For this review, take the finished solid that the model builds, in its own axes (mm). Face numbers are marked on the shaded views. A direction names the side the tool comes from. Round coordinates to 2 decimals unless told otherwise and drop trailing zeros. Order: outer loops, then holes, each group sorted by start corner. A loop starts at its lowest first (then second) coordinate and runs counter-clockwise, first axis right, second up.
```python
from build123d import *

# Parameters (mm, degrees)
SKETCH1_W               = 69.85
SKETCH1_H               = 29.464
BOSS_EXTRUDE1_DEPTH     = 16.764
SKETCH2_W               = 25.4
SKETCH2_H               = 6.35
CUT_EXTRUDE1_DEPTH      = 69.85
SKETCH3_W               = 25.4
SKETCH3_H               = 6.35
CUT_EXTRUDE2_DEPTH      = 50.8
SKETCH5_W               = 61.722
SKETCH5_H               = 17.1196
CUT_EXTRUDE3_DEPTH      = 1.016
SKETCH5_3_R             = 0.81915
CUT_EXTRUDE4_DEPTH      = 42.446581825
SKETCH7_W               = 69.85
SKETCH7_H               = 7.62
BOSS_EXTRUDE2_DEPTH     = 25.4
CUT_EXTRUDE9_DEPTH      = 74.328616651
CUT_EXTRUDE9_DEPTH_BACK = 74.328616651
SKETCH13_R              = 2.7051
CUT_EXTRUDE12_DEPTH     = 4.064
SKETCH17_W              = 1.905
SKETCH17_H              = 6.477
CUT_EXTRUDE13_DEPTH     = 25.4
FILLET1_R               = 7.62


with BuildPart() as part:
    # Sketch1 → Boss-Extrude1 (new body)
    with BuildSketch(Plane(origin=(0, 0, 0), x_dir=(1, 0, 0), z_dir=(0, 1, 0))):
        Rectangle(SKETCH1_W, SKETCH1_H)
    extrude(amount=BOSS_EXTRUDE1_DEPTH)

    # Sketch2 → Cut-Extrude1 (cut)
    with BuildSketch(Plane.ZY.offset(34.925)):
        with Locations((-2.032, 7.239)):
            Rectangle(SKETCH2_W, SKETCH2_H)
    extrude(amount=-CUT_EXTRUDE1_DEPTH, mode=Mode.SUBTRACT)

    # Sketch3 → Cut-Extrude2 (cut)
    with BuildSketch(Plane.ZY.offset(34.925)):
        with Locations((-2.032, 13.589)):
            Rectangle(SKETCH3_W, SKETCH3_H)
    cut_extrude2 = extrude(amount=-CUT_EXTRUDE2_DEPTH, mode=Mode.SUBTRACT)

    # Mirror1: Cut-Extrude2 across plane
    add(cut_extrude2.mirror(Plane(origin=(0, 0, 0), x_dir=(0, 0, 1), z_dir=(1, 0, 0))), mode=Mode.SUBTRACT)

    # Sketch5 → Cut-Extrude3 (cut)
    with BuildSketch(Plane.XZ):
        with Locations((0, 6.1722)):
            Rectangle(SKETCH5_W, SKETCH5_H)
    extrude(amount=-CUT_EXTRUDE3_DEPTH, mode=Mode.SUBTRACT)

    # Sketch5<3> → Cut-Extrude4 (cut, through all)
    with BuildSketch(Plane.XZ):
        with Locations(Location((-27.9908, 0.1524, 0), (0, 0, 270))):
            Circle(SKETCH5_3_R)
        with Locations(Location((27.9908, 0.1524, 0), (0, 0, 270))):
            Circle(SKETCH5_3_R)
    extrude(amount=-CUT_EXTRUDE4_DEPTH, mode=Mode.SUBTRACT)

    # Sketch7 → Boss-Extrude2 (add)
    with BuildSketch(Plane(origin=(0, 0, 10.668), x_dir=(-1, 0, 0), z_dir=(0, 0, -1))):
        with Locations((0, 12.954)):
            Rectangle(SKETCH7_W, SKETCH7_H)
    extrude(amount=BOSS_EXTRUDE2_DEPTH)

    # Sketch8 → Cut-Extrude9 (cut, two sides: drawn at the far end of the back side and taken through both)
    with BuildSketch(Plane.ZY.offset(34.925).offset(-CUT_EXTRUDE9_DEPTH_BACK)):
        Polygon((-14.732, 10.287), (10.668, 10.668), (10.668, 9.144), (-14.732, 9.144), align=None)
    extrude(amount=CUT_EXTRUDE9_DEPTH + CUT_EXTRUDE9_DEPTH_BACK, mode=Mode.SUBTRACT)

    # Sketch13 → Cut-Extrude12 (cut)
    with BuildSketch(Plane.XY.offset(14.732)):
        with Locations((-19.685, 8.382)):
            Circle(SKETCH13_R)
        with Locations((19.685, 8.382)):
            Circle(SKETCH13_R)
    extrude(amount=-CUT_EXTRUDE12_DEPTH, mode=Mode.SUBTRACT)

    # Sketch17 → Cut-Extrude13 (cut)
    with BuildSketch(Plane(origin=(0, 0, -14.732), x_dir=(-1, 0, 0), z_dir=(0, 0, -1))):
        with Locations((-33.9725, 13.5255)):
            Rectangle(SKETCH17_W, SKETCH17_H)
        with Locations((33.9725, 13.5255)):
            Rectangle(SKETCH17_W, SKETCH17_H)
    extrude(amount=-CUT_EXTRUDE13_DEPTH, mode=Mode.SUBTRACT)

    # Fillet1
    # the kernel refuses this fillet: 7.62 mm, written as the material it adds along each edge
    with BuildSketch(Plane(origin=(-33.02, 16.764, 10.668), x_dir=(0, 0, -1), z_dir=(0, -1, 0))) as fillet1_piece_1_section:
        with BuildLine():
            CenterArc((5.040156248, -7.62), FILLET1_R, 90, 41.409622109)
            Line((0, -1.905), (-0.100803125, -1.7907))
            ThreePointArc((-0.100803125, -1.7907), (-0.1524, -0.9525), (-0.1524, 0))
            Line((-0.1524, 0), (0, 0.1524))
            Line((0, 0.1524), (5.040156248, 0.1524))
            Line((5.040156248, 0.1524), (5.040156248, 0))
        make_face()
    fillet1_piece_1 = extrude(amount=18.696390619, mode=Mode.PRIVATE)
    fillet1_piece_1 = split(fillet1_piece_1, bisect_by=Plane(origin=(-33.474653721, 10.647897951, 9.327863423), z_dir=(0, 0.9998875189808162, -0.014998312784712252)), keep=Keep.TOP, mode=Mode.PRIVATE)
    add(fillet1_piece_1)
    with BuildSketch(Plane(origin=(33.02, -1.932390619, 10.668), x_dir=(0, 0, -1), z_dir=(0, 1, 0))) as fillet1_piece_2_section:
        with BuildLine():
            CenterArc((5.040156248, -7.62), FILLET1_R, 90, 41.409622109)
            Line((0, -1.905), (-0.100803125, -1.7907))
            ThreePointArc((-0.100803125, -1.7907), (-0.1524, -0.9525), (-0.1524, 0))
            Line((-0.1524, 0), (0, 0.1524))
            Line((0, 0.1524), (5.040156248, 0.1524))
            Line((5.040156248, 0.1524), (5.040156248, 0))
        make_face()
    fillet1_piece_2 = extrude(amount=18.696390619, mode=Mode.PRIVATE)
    fillet1_piece_2 = split(fillet1_piece_2, bisect_by=Plane(origin=(33.474653721, 10.647897951, 9.327863423), z_dir=(0, 0.9998875189808162, -0.014998312784712252)), keep=Keep.TOP, mode=Mode.PRIVATE)
    add(fillet1_piece_2)


solid = part.part
```
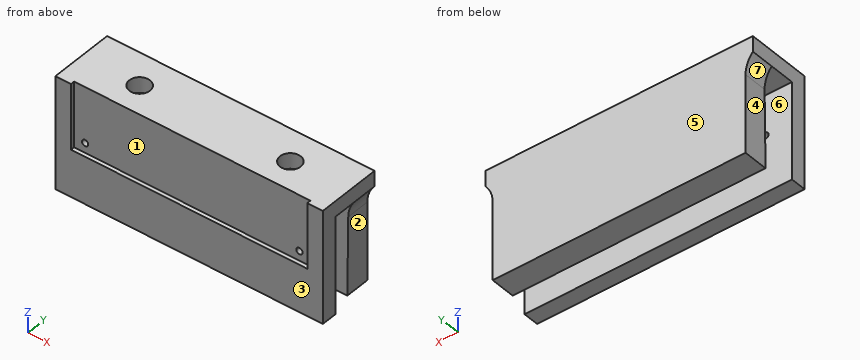
Q1. Wall thickness on line 1 (Z direction, x = -26.5, y = 9.75); line 2 (Z direction, x = -28, y = 2.5); line 3 (Y direction, x = 11, z = 5.5): over which ranges is each line inside the solid? List them lowest first.
Q2. Mouldability with a two-part tool opening along X and no side actions: class the marked faces 1, 2, 3 and 4 as +X half, -X half, draft (parallel to the pull), parting line (faces both ways), or undercut.
Q3. Clearance check with flat-ended pins moving along their axes: pin 1 (1.9 mm diameter, centred on y = 12, z = -9.5, fed in from +X); pin 2 (3 mm diameter, centred on y = 12.5, z = -5, fed in from -X); pin 3 (2 mm diameter, centred on x = -10, y = 8, fed in from -Z). State where each tip first meets the part, or that it passes through.
Q4. Take a section at C-C, the plane y = 15. State the section outline as (x, z) points (3 decimals), plus the area to 3 significant figures.
Q5. Take a section at B-B, the plane x = -19. State the section outline as (y, z) points, plus the area to 3 significant figures.
Q6. Take a section at A-A, the plane z = -3.5. State the section outline as (x, y) points (3 decimals), plus the area to 3 significant figures.
Q7. Tool access review of the marked faces 5, 6 and 7: name each direction out of +Z, -Z, +X, -X, +Y, -Y from which nothing blocks a thin tool from reaching the whole face with its end or side.
Q8. Take a section at D-D, the plane x = -2. State the section outline as (y, z) points.
Working result:
1. line 1: z = 10.67 to 14.73
1. line 2: z = -14.73 to -0.67, 0.97 to 14.73
1. line 3: y = 1.02 to 4.06, 10.59 to 16.76
2. face 1: undercut
2. face 2: +X half
2. face 3: draft
2. face 4: -X half
3. pin 1: stops at x = 33.02
3. pin 2: stops at x = -33.02
3. pin 3: stops at z = 10.67
4. outline: (-34.925, 10.668) arc R7.62 cw to (-33.02, 5.628) - (-33.02, -14.732) - (33.02, -14.732) - (33.02, 5.628) arc R7.62 cw to (34.925, 10.668) - (34.925, 14.732) - (-34.925, 14.732) - close
4. area: 1,970 mm2
5. outline: (0, -14.73) - (4.06, -14.73) - (4.06, 10.67) - (5.77, 10.67) - (5.77, 14.73) - (1.02, 14.73) - (1.02, -2.39) - (0, -2.39) - close; (10.29, -14.73) - (16.76, -14.73) - (16.76, 14.73) - (11, 14.73) - (11, 10.67) - (10.67, 10.67) - close
5. area: 292 mm2
6. outline: (-34.925, 0) - (34.925, 0) - (34.925, 4.064) - (-34.925, 4.064) - close; (-33.02, 10.455) - (33.02, 10.455) - (33.02, 16.764) - (-33.02, 16.764) - close
6. area: 700 mm2
7. face 5: +Z, -Z, +X, -X, +Y
7. face 6: -Z, +X, -X
7. face 7: -Z, -X, +Y
8. outline: (0, -14.73) - (4.06, -14.73) - (4.06, 10.67) - (10.67, 10.67) - (10.29, -14.73) - (16.76, -14.73) - (16.76, 14.73) - (1.02, 14.73) - (1.02, -2.39) - (0, -2.39) - close
